Check sheet for the modelled part. Datum: model origin and axes. Units: mm. Face numbers are marked on the shaded views. A direction names the side the tool comes from. Coordinates: 2 decimals unless noted, no trailing zeros. Order: outer loops, then holes, each group sorted by start corner. A loop starts at its lowest first (then second) coordinate and runs counter-clockwise, first axis right, second up.
1. Cross-section at A-A (z = -28.5). Enter the section's corners in (x, y), then the cut area to 3 significant figures.
2. Cross-section at B-B (x = 23.5). Enter the section's corners in (y, z).
3. Set-up check for the marked faces 1, 2, 3 and 4: record each of +Z, -Z, +X, -X, +Y, -Y from which the full face is reachable in a straight line by a thin tool's end or side.
4. Cross-section at D-D (x = 38.1). Enter the section's corners in (y, z), then the cut area to 3 significant figures.
5. Draft check along Z on the marked faces 5, 6 and 7. Enter one of: released by +Z, released by -Z, zero draft, split by the parting line, or undercut.
6. Thickness scan on line 1 (X direction, y = -27, z = -8); line 2 (Y direction, x = 38, z = 1); line 3 (X direction, y = 0, z = -1.75). Record the ranges inside material, lowest first.
7. Cross-section at C-C (y = 29). Enter the section's corners in (x, z), then the cut area to 3 significant figures.
8. Gauge pin test, flat ends, axial feed: pin 1 Ø23 at (x, y) = (38.1, 0) entering from +Z; pin 2 Ø1 at (x, z) = (64.5, -65.5) entering from +Y. Record the tip position at first contact, or that the pin passes through.
```python
from build123d import *

# Parameters (mm, degrees)
F1_DEPTH = 38.1
F2_DEPTH = 12.7
F3_R     = 12.7
F4_DEPTH = 25.4


with BuildPart() as f1:
    # F0 (on Front) → F1 (new body, symmetric)
    with BuildSketch(Plane.XZ):
        with BuildLine():
            ThreePointArc((0, -6.35), (1.8598719395, -1.8598719395), (6.35, 0))
            Line((6.35, 0), (44.45, 0))
            Line((44.45, 0), (88.9, 0))
            Line((88.9, 0), (88.9, 6.35))
            ThreePointArc((88.9, 6.35), (87.0401280605, 10.8401280605), (82.55, 12.7))
            Line((82.55, 12.7), (-31.75, 12.7))
            ThreePointArc((-31.75, 12.7), (-36.2401280605, 10.8401280605), (-38.1, 6.35))
            Line((-38.1, 6.35), (-38.1, -69.85))
            ThreePointArc((-38.1, -69.85), (-36.2401280605, -74.3401280605), (-31.75, -76.2))
            Line((-31.75, -76.2), (0, -76.2))
            Line((0, -76.2), (0, -44.45))
            Line((0, -44.45), (0, -6.35))
        make_face()
        with BuildLine():
            ThreePointArc((-25.4, -3.81), (-24.2840768363, -1.1159231637), (-21.59, 0))
            Line((-21.59, 0), (-16.51, 0))
            ThreePointArc((-16.51, 0), (-13.8159231637, -1.1159231637), (-12.7, -3.81))
            Line((-12.7, -3.81), (-12.7, -59.69))
            ThreePointArc((-12.7, -59.69), (-13.8159231637, -62.3840768363), (-16.51, -63.5))
            Line((-16.51, -63.5), (-21.59, -63.5))
            ThreePointArc((-21.59, -63.5), (-24.2840768363, -62.3840768363), (-25.4, -59.69))
            Line((-25.4, -59.69), (-25.4, -3.81))
        make_face(mode=Mode.SUBTRACT)
    extrude(amount=F1_DEPTH, both=True)

    # F0 (on Front) → F2 (join, symmetric)
    with BuildSketch(Plane.XZ):
        with BuildLine():
            ThreePointArc((0, -6.35), (1.8598719395, -1.8598719395), (6.35, 0))
            Line((6.35, 0), (44.45, 0))
            Line((44.45, 0), (88.9, 0))
            Line((88.9, 0), (88.9, 6.35))
            ThreePointArc((88.9, 6.35), (87.0401280605, 10.8401280605), (82.55, 12.7))
            Line((82.55, 12.7), (-31.75, 12.7))
            ThreePointArc((-31.75, 12.7), (-36.2401280605, 10.8401280605), (-38.1, 6.35))
            Line((-38.1, 6.35), (-38.1, -69.85))
            ThreePointArc((-38.1, -69.85), (-36.2401280605, -74.3401280605), (-31.75, -76.2))
            Line((-31.75, -76.2), (0, -76.2))
            Line((0, -76.2), (0, -44.45))
            Line((0, -44.45), (0, -6.35))
        make_face()
        with BuildLine():
            ThreePointArc((-25.4, -3.81), (-24.2840768363, -1.1159231637), (-21.59, 0))
            Line((-21.59, 0), (-16.51, 0))
            ThreePointArc((-16.51, 0), (-13.8159231637, -1.1159231637), (-12.7, -3.81))
            Line((-12.7, -3.81), (-12.7, -59.69))
            ThreePointArc((-12.7, -59.69), (-13.8159231637, -62.3840768363), (-16.51, -63.5))
            Line((-16.51, -63.5), (-21.59, -63.5))
            ThreePointArc((-21.59, -63.5), (-24.2840768363, -62.3840768363), (-25.4, -59.69))
            Line((-25.4, -59.69), (-25.4, -3.81))
        make_face(mode=Mode.SUBTRACT)
        with BuildLine():
            Line((88.9, 0), (44.45, 0))
            ThreePointArc((44.45, 0), (48.9401280605, -1.8598719395), (50.8, -6.35))
            Line((50.8, -6.35), (50.8, -44.45))
            ThreePointArc((50.8, -44.45), (48.9401280605, -48.9401280605), (44.45, -50.8))
            Line((44.45, -50.8), (6.35, -50.8))
            ThreePointArc((6.35, -50.8), (1.8598719395, -48.9401280605), (0, -44.45))
            Line((0, -44.45), (0, -76.2))
            Line((0, -76.2), (82.55, -76.2))
            ThreePointArc((82.55, -76.2), (87.0401280605, -74.3401280605), (88.9, -69.85))
            Line((88.9, -69.85), (88.9, 0))
        make_face()
    extrude(amount=F2_DEPTH, both=True)

    # F3 (on face) → F4 (cut)
    with BuildSketch(Plane.XY.offset(12.7)):
        with Locations((38.1, 0)):
            Circle(F3_R)
    extrude(amount=-F4_DEPTH, mode=Mode.SUBTRACT)


solid = f1.part
```
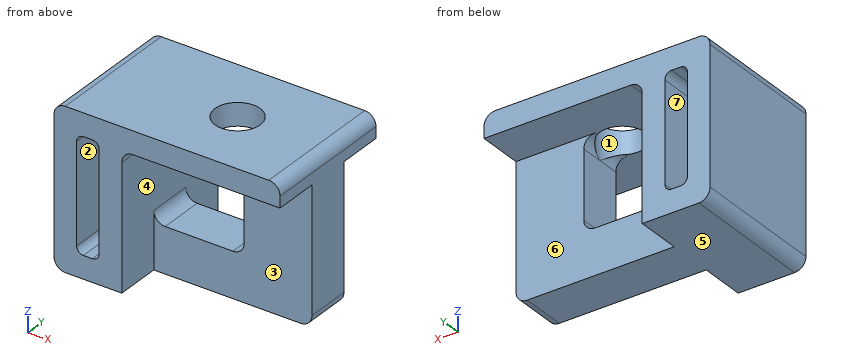
Data:
1. outline: (-38.1, -38.1) - (-25.4, -38.1) - (-25.4, 38.1) - (-38.1, 38.1) - close; (-12.7, -38.1) - (0, -38.1) - (0, 38.1) - (-12.7, 38.1) - close; (50.8, -12.7) - (88.9, -12.7) - (88.9, 12.7) - (50.8, 12.7) - close
1. area: 2,900 mm2
2. outline: (-38.1, 0) - (38.1, 0) - (38.1, 12.7) - (-38.1, 12.7) - close; (-12.7, -76.2) - (12.7, -76.2) - (12.7, -50.8) - (-12.7, -50.8) - close
3. face 1: +Z
3. face 2: +Y, -Y
3. face 3: -Z, +X, -Y
3. face 4: none
4. outline: (-38.1, 0) - (-12.7, 0) - (-12.7, 12.7) - (-38.1, 12.7) - close; (-12.7, -76.2) - (12.7, -76.2) - (12.7, -50.8) - (-12.7, -50.8) - close; (12.7, 0) - (38.1, 0) - (38.1, 12.7) - (12.7, 12.7) - close
4. area: 1,290 mm2
5. face 5: released by -Z
5. face 6: zero draft
5. face 7: undercut
6. line 1: x = -38.1 to -25.4, -12.7 to 0
6. line 2: y = -38.1 to -12.7, 12.7 to 38.1
6. line 3: x = -38.1 to -24.8, -13.3 to 1.97, 50.8 to 88.9
7. outline: (-38.1, -69.85) arc R6.35 ccw to (-31.75, -76.2) - (0, -76.2) - (0, -6.35) arc R6.35 cw to (6.35, 0) - (88.9, 0) - (88.9, 6.35) arc R6.35 ccw to (82.55, 12.7) - (-31.75, 12.7) arc R6.35 ccw to (-38.1, 6.35) - close; hole (-25.4, -59.69) arc R3.81 ccw to (-21.59, -63.5) - (-16.51, -63.5) arc R3.81 ccw to (-12.7, -59.69) - (-12.7, -3.81) arc R3.81 ccw to (-16.51, 0) - (-21.59, 0) arc R3.81 ccw to (-25.4, -3.81) - close
7. area: 3,700 mm2
8. pin 1: stops at z = -48.16
8. pin 2: stops at y = 12.7
